Build history of the part. All positions in model axes, mm. A direction names the side the tool comes from. Round coordinates to 2 decimals unless told otherwise and drop trailing zeros. Write each loop counter-clockwise with the first axis right and the second up, starting at its lowest first coordinate (ties: lowest second). Pieces come first, ordered by that corner, then holes. Notation, with made-up numbers: (-9, 2) - (28, 2) arc R10 ccw to (28, 18) - close; hole circle Ø5 at (32, 77.25). An arc over 180 degrees is marked (long way). Answer as a JSON object with one key per item and string values. Group by question number.
Item 1: Slice it at A-A, the plane x = 13. List the corners of the cut face in (y, z), then the cut area to 3 significant figures.
Item 2: Flat gauge pin, fed straight in: pin 1 (2 mm diameter, centred on x = 1, y = -11.5, fed in from +Z). Where does the tip first touch, or does it go through?
Item 3: Which spindle directions (+Z, -Z, +X, -X, +Y, -Y) get a long thin tool onto all of the face, cutting with end or side? Do faces 1 (the flat face through (0, 0, 0)), 2 (the flat face through (4, 0, 1)). Say none if no direction does.
Item 4: Probe line 1 (Z direction, x = -2.5, y = 16.5); line 2 (X direction, y = -7.5, z = 1.05); line 3 (X direction, y = 12.5, z = 1.55). List the from-to ranges inside material, lowest first. Write a range as from..to.
from build123d import *

# Parameters (mm, degrees)
EXTRUDE001_DEPTH = 1
EXTRUDE_DEPTH    = 0.6
CYLINDER_R       = 20
CYLINDER_DEPTH   = 1


with BuildPart() as body:
    # path4_7_6_1_6 → Extrude001 (new body)
    with BuildSketch(Plane(origin=(-0.182391, 4.245198, 1), x_dir=(0, -1, 0), z_dir=(0, 0, -1))):
        with BuildLine():
            add(Edge.make_bspline(
                [(-5.179264, 6.636207), (-10.812113, -0.699558)],
                knots=[0, 0, 32.771748, 32.771748], degree=1))
            add(Edge.make_bspline(
                [(-10.812113, -0.699558), (-9.469887, -6.636207)],
                knots=[0, 0, 21.566306, 21.566306], degree=1))
            add(Edge.make_bspline(
                [(-9.469887, -6.636207), (10.812113, -1.892574)],
                knots=[0, 0, 73.804763, 73.804763], degree=1))
            add(Edge.make_bspline(
                [(10.812113, -1.892574), (9.768057, 2.72503)],
                knots=[0, 0, 16.774602, 16.774602], degree=1))
            add(Edge.make_bspline(
                [(9.768057, 2.72503), (-6.421163, -0.923188)],
                knots=[0, 0, 58.801858, 58.801858], degree=1))
            add(Edge.make_bspline(
                [(-6.421163, -0.923188), (-3.132877, 4.49797)],
                knots=[0, 0, 22.466297, 22.466297], degree=1))
            add(Edge.make_bspline(
                [(-3.132877, 4.49797), (-5.179264, 6.636207)],
                knots=[0, 0, 10.487087, 10.487087], degree=1))
        make_face()
    extrude(amount=EXTRUDE001_DEPTH)


with BuildPart() as body_1:
    # Extrude001 placement: moved
    add(body.part.moved(Location((0, 0, 1))))


with BuildPart() as fusion:
    # path6_7_2_1_0_9 → Extrude (new body)
    with BuildSketch(Plane(origin=(-2.209018, -10.301053, 1), x_dir=(0, 1, 0), z_dir=(0, 0, 1))):
        with BuildLine():
            add(Edge.make_bspline(
                [(5.102704, -0.748152), (0.480762, 1.277563)],
                knots=[0, 0, 17.880845, 17.880845], degree=1))
            add(Edge.make_bspline(
                [(0.480762, 1.277563), (-0.416615, 5.870839)],
                knots=[0, 0, 16.583084, 16.583084], degree=1))
            add(Edge.make_bspline(
                [(-0.416615, 5.870839), (-0.481689, 6.203856), (-0.809722, 6.416714), (-1.140362, 6.340474)],
                knots=[0, 0, 0, 0, 1, 1, 1, 1], degree=3))
            add(Edge.make_bspline(
                [(-1.140362, 6.340474), (-2.696993, 5.981634)],
                knots=[0, 0, 5.660276, 5.660276], degree=1))
            add(Edge.make_bspline(
                [(-2.696993, 5.981634), (-3.498944, 5.81621), (-3.220876, 4.610113), (-2.427448, 4.812506)],
                knots=[0, 0, 0, 0, 1, 1, 1, 1], degree=3))
            add(Edge.make_bspline(
                [(-2.427448, 4.812506), (-1.475501, 5.031338)],
                knots=[0, 0, 3.461016, 3.461016], degree=1))
            add(Edge.make_bspline(
                [(-1.475501, 5.031338), (-0.63655, 0.739027)],
                knots=[0, 0, 15.496767, 15.496767], degree=1))
            add(Edge.make_bspline(
                [(-0.63655, 0.739027), (-0.598809, 0.545987), (-0.468854, 0.383697), (-0.288734, 0.30467)],
                knots=[0, 0, 0, 0, 1, 1, 1, 1], degree=3))
            add(Edge.make_bspline(
                [(-0.288734, 0.30467), (4.397148, -1.74916)],
                knots=[0, 0, 18.12834, 18.12834], degree=1))
            add(Edge.make_bspline(
                [(4.397148, -1.74916), (0.091606, -4.999124)],
                knots=[0, 0, 19.114151, 19.114151], degree=1))
            add(Edge.make_bspline(
                [(0.091606, -4.999124), (-3.255375, -2.197298)],
                knots=[0, 0, 15.466244, 15.466244], degree=1))
            add(Edge.make_bspline(
                [(-3.255375, -2.197298), (-3.503985, -1.989464), (-3.872691, -2.016549), (-4.088261, -2.258481)],
                knots=[0, 0, 0, 0, 1, 1, 1, 1], degree=3))
            add(Edge.make_bspline(
                [(-4.088261, -2.258481), (-5.046273, -3.333903)],
                knots=[0, 0, 5.103247, 5.103247], degree=1))
            add(Edge.make_bspline(
                [(-5.046273, -3.333903), (-5.57838, -3.931421), (-4.682104, -4.729582), (-4.149997, -4.132064)],
                knots=[0, 0, 0, 0, 1, 1, 1, 1], degree=3))
            add(Edge.make_bspline(
                [(-4.149997, -4.132064), (-3.57949, -3.490999)],
                knots=[0, 0, 3.040732, 3.040732], degree=1))
            add(Edge.make_bspline(
                [(-3.57949, -3.490999), (-0.312988, -6.22558)],
                knots=[0, 0, 15.094642, 15.094642], degree=1))
            add(Edge.make_bspline(
                [(-0.312988, -6.22558), (-0.098751, -6.404963), (0.210946, -6.412733), (0.43391, -6.244319)],
                knots=[0, 0, 0, 0, 1, 1, 1, 1], degree=3))
            add(Edge.make_bspline(
                [(0.43391, -6.244319), (5.343033, -2.538499)],
                knots=[0, 0, 21.794246, 21.794246], degree=1))
            add(Edge.make_bspline(
                [(5.343033, -2.538499), (5.102704, -0.748152)],
                knots=[0, 0, 6.40065, 6.40065], degree=1))
        make_face()
    extrude(amount=EXTRUDE_DEPTH)

    # Fusion: union Body
    add(body_1.part)


with BuildPart() as bit_1_coin:
    # Cylinder → Cylinder (new body)
    with BuildSketch(Plane.XY):
        Circle(CYLINDER_R)
    extrude(amount=CYLINDER_DEPTH)

    # Fusion001: union Fusion
    add(fusion.part)


solid = bit_1_coin.part
Geometry says:
{
 "1": {"outline": "(-15.2, 0) - (15.2, 0) - (15.2, 1) - (-15.2, 1) - close", "area": "30.4 mm^2"},
 "2": {"pin 1": "stops at z = 1.6"},
 "3": {"face 1": "-Z, +X, -X, +Y, -Y", "face 2": "+Z"},
 "4": {"line 1": "z = 0..1", "line 2": "x = -2.47..-1.16, 0.74..2.25", "line 3": "x = -2.81..6.17"}
}
